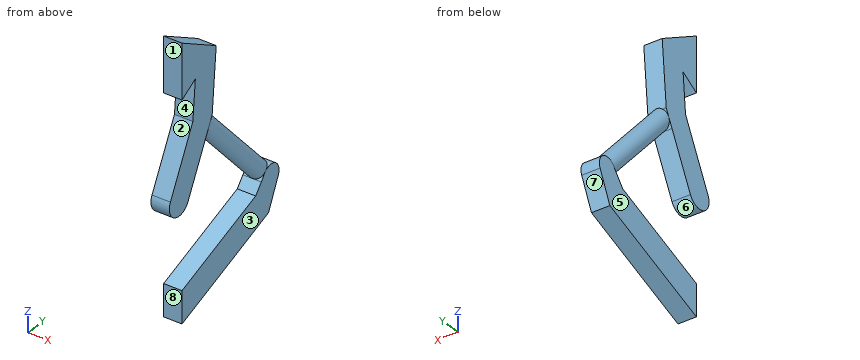
from build123d import *

# Parameters (mm, degrees)
EXTRUDE_1_DEPTH = 10


with BuildPart() as part:
    # Sketch 1 → Revolve 1 (revolve)
    with BuildSketch(Plane(origin=(0, 0, 0), x_dir=(0, 0, -1), z_dir=(1, 0, 0)), mode=Mode.PRIVATE) as revolve_1_sk:
        with BuildLine():
            ThreePointArc((40.921436703, 123.884958945), (38.783143174, 125.157716321), (36.942224664, 126.832001121))
            Line((36.942224664, 126.832001121), (-57.525228671, 41.916313142))
            Line((-57.525228671, 41.916313142), (-47.978183475, 37.051850647))
            Line((-47.978183475, 37.051850647), (44.904364471, 120.542885724))
            Line((44.904364471, 120.542885724), (40.921436703, 123.884958945))
        make_face()
        Polygon((-47.978183475, 37.051850647), (-57.525228671, 41.916313142), (-69.478316775, 31.171822167), (-62.793238575, 23.73477104), align=None)
        with BuildLine():
            Line((46.158922046, 135.116782508), (36.942224664, 126.832001121))
            ThreePointArc((36.942224664, 126.832001121), (38.783143174, 125.157716321), (40.921436703, 123.884958945))
            Line((40.921436703, 123.884958945), (44.904364471, 120.542885724))
            Line((44.904364471, 120.542885724), (52.844000246, 127.679731381))
            Line((52.844000246, 127.679731381), (46.158922046, 135.116782508))
        make_face()
    revolve(revolve_1_sk.sketch.rotate(Axis((0, 135.116782508, -46.158922046), (0, -0.6685078200290915, 0.7437051126353456)), 180), axis=Axis((0, 135.116782508, -46.158922046), (0, -0.6685078200290915, 0.7437051126353456)))

    # Sketch 1_3 → Extrude 1 (add, symmetric)
    with BuildSketch(Plane(origin=(0, 0, 0), x_dir=(0, 0, -1), z_dir=(1, 0, 0))):
        with BuildLine():
            Line((95.882133508, 0), (131, 0))
            Line((131, 0), (83.117179934, 131.55696691))
            Line((83.117179934, 131.55696691), (51.396407388, 146.348606071))
            ThreePointArc((51.396407388, 146.348606071), (36.199855859, 142.492561379), (36.942224664, 126.832001121))
            Line((36.942224664, 126.832001121), (46.158922046, 135.116782508))
            Line((46.158922046, 135.116782508), (52.844000246, 127.679731381))
            Line((52.844000246, 127.679731381), (44.904364471, 120.542885724))
            Line((44.904364471, 120.542885724), (55.131576148, 111.961236177))
            Line((55.131576148, 111.961236177), (95.882133508, 0))
        make_face()
        with BuildLine():
            Line((46.158922046, 135.116782508), (36.942224664, 126.832001121))
            ThreePointArc((36.942224664, 126.832001121), (38.783143174, 125.157716321), (40.921436703, 123.884958945))
            Line((40.921436703, 123.884958945), (44.904364471, 120.542885724))
            Line((44.904364471, 120.542885724), (52.844000246, 127.679731381))
            Line((52.844000246, 127.679731381), (46.158922046, 135.116782508))
        make_face()
        with BuildLine():
            Line((-69.478316775, 31.171822167), (-57.525228671, 41.916313142))
            Line((-57.525228671, 41.916313142), (-65.266371134, 45.860622235))
            Line((-65.266371134, 45.860622235), (-135, 51.961524227))
            Line((-135, 51.961524227), (-165, 0))
            Line((-165, 0), (-105, 0))
            Line((-105, 0), (-116.688381169, 20.244870042))
            Line((-116.688381169, 20.244870042), (-73.690262417, 16.483022099))
            Line((-73.690262417, 16.483022099), (-6.714557667, -17.64280397))
            ThreePointArc((-6.714557667, -17.64280397), (13.460397692, -11.087563603), (6.905157326, 9.087391756))
            Line((6.905157326, 9.087391756), (-47.978183475, 37.051850647))
            Line((-47.978183475, 37.051850647), (-62.793238575, 23.73477104))
            Line((-62.793238575, 23.73477104), (-69.478316775, 31.171822167))
        make_face()
        Polygon((-47.978183475, 37.051850647), (-57.525228671, 41.916313142), (-69.478316775, 31.171822167), (-62.793238575, 23.73477104), align=None)
    extrude(amount=EXTRUDE_1_DEPTH, both=True)


solid = part.part
Read the model definition and answer for the solid it produces. Units are mm, in the model's axes. Face numbers are marked on the shaded views. A direction names the side the tool comes from. Give positions to 0.01 mm unless a question says otherwise; leave off trailing zeros. Loops run counter-clockwise (first coordinate to the right, second up) from the corner with the lowest first, then second, coordinate; pieces in that order, holes last. Notation, with made-up numbers: (63.5, 45.25) -> (70.5, 45.25) arc R10 ccw to (70.5, 51.25) -> close; hole circle Ø10 at (30, -21.75). An arc over 180 degrees is marked (long way). Use a Markdown table: item, result.
Q1. A tool of negligible diameter and unlimited length cuts with its end or side. For the marked faces 1, 2, 3 and 4, from which of +Z, -Z, +X, -X, +Y, -Y can it reach the whole face along a straight path? Write none if from no direction.
Solved:
| item | result |
|---|---|
| face 1 | +Z, +X, -X, -Y |
| face 2 | +X, -X, -Y |
| face 3 | +Z, -Z, +X, +Y, -Y |
| face 4 | +X, -X |
Q2. Section B-B, the plane y = -9 is taken. Determine the outline of the cut face in (x, z).
Solved:
| item | result |
|---|---|
| outline | (-10, -14.33) -> (10, -14.33) -> (10, 23.68) -> (-10, 23.68) -> close |
Q3. Find the intervals of material crossed by line 1 along Z through (x, y) = (7.75, 8.5); line 2 along Z through (x, y) = (-2.75, 100.5); line 3 along Z through (x, y) = (0.5, 15), in increasing order.
Solved:
| item | result |
|---|---|
| line 1 | z = -127.91 to -92.79, -7.95 to 58.02, 109.91 to 160.09 |
| line 2 | z = -94.42 to -59.3, -22.03 to 6.73 |
| line 3 | z = -125.54 to -90.42, 4.7 to 70.78, 113.66 to 156.34 |
Q4. Determine the mould class of the marked faces 5, 6, 7 and 8 for opening direction Y: pulls with the +Y half, pulls with the -Y half, needs draft (parallel to the pull), parting line crosses it, or undercut.
Solved:
| item | result |
|---|---|
| face 5 | needs draft |
| face 6 | undercut |
| face 7 | pulls with the +Y half |
| face 8 | pulls with the -Y half |
Q5. Section A-A, the plane z = -109 is taken. Determine the outline of the cut face in (x, y), then the cut area to 3 significant figures.
Solved:
| item | result |
|---|---|
| outline | (-10, 0) -> (10, 0) -> (10, 60.44) -> (-10, 60.44) -> close |
| area | 1,210 mm^2 |
Q6. Each of these flat-tipped pins is pushed along its axis until it touches: pin 1 (2 mm diameter, centred on x = 4.5, z = 74, fed in from -Y); pin 2 (6 mm diameter, centred on x = -0.5, z = 129.5, fed in from -Y); pin 3 (6 mm diameter, centred on x = 5, y = 97, fed in from -Z). Where does it stop, or does it pass through?
Solved:
| item | result |
|---|---|
| pin 1 | stops at y = 16.13 |
| pin 2 | stops at y = 0 |
| pin 3 | stops at z = -96.79 |
